Design review of the part shown in the three views and the two pictorial views. Dimensions are in mm from the part's minimum x, y and z. A direction names the side the tool comes from. Give positions to 0.01 mm unless a question says otherwise; leave off trailing zeros. Order: outer loops, then holes, each group sorted by start corner. A loop starts at its lowest first (then second) coordinate and runs counter-clockwise, first axis right, second up. Notation, with made-up numbers: (-3, -7.5) -> (22, -7.5) arc R20 cw to (22, 9.5) -> close; hole circle Ø1 at (61, 77.5). An arc over 180 degrees is marked (long way). Use one line per item in the form item = value.
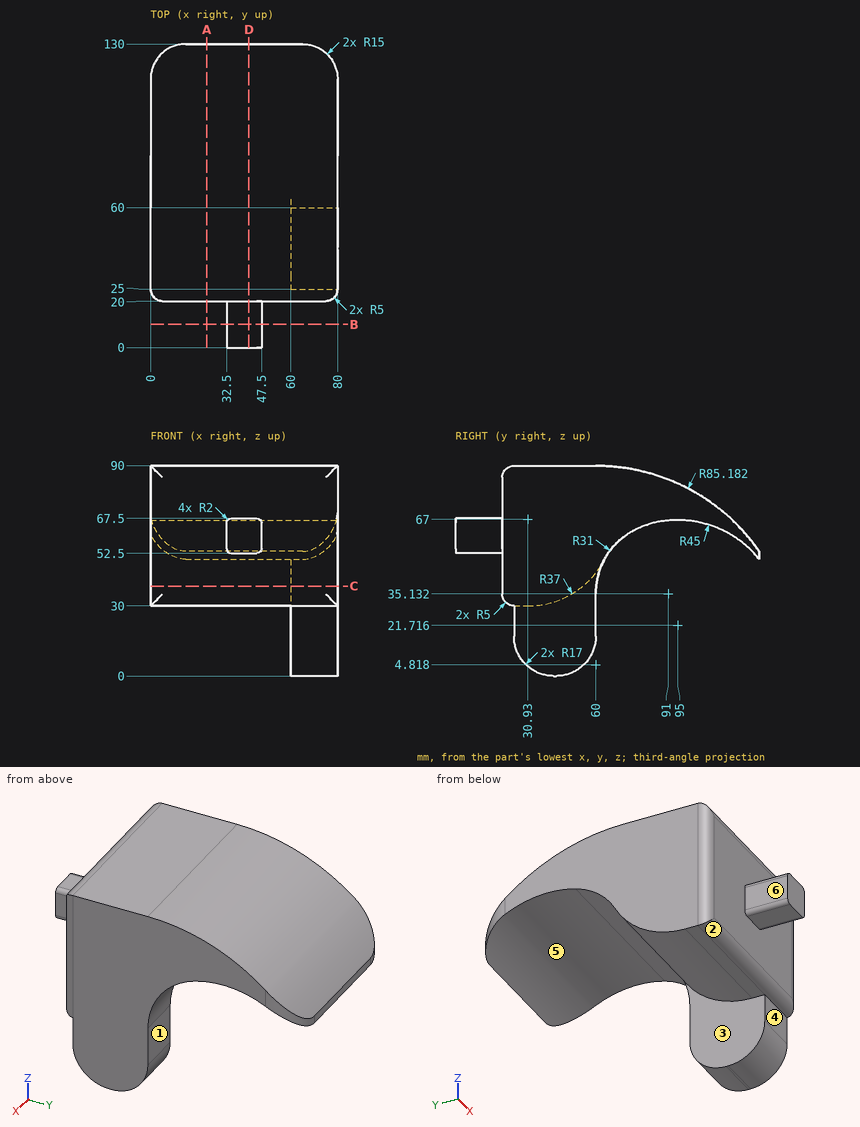
1. Add section C-C on z = 38.5. Give the boundary of the cut face in (x, y) (1 decimal), then the cut area to 3 significant figures.
Values:
outline = (0, 25) arc R5 ccw to (5, 20) -> (75, 20) arc R5 ccw to (80, 25) -> (80, 60.2) -> (60, 60.2) -> (60, 54.5) -> (0, 54.5) -> close
area = 2,860 mm^2
2. Add section B-B on y = 10. Give the boundary of the cut face in (x, z), then the cut area to 3 significant figures.
Values:
outline = (32.5, 54.5) arc R2 ccw to (34.5, 52.5) -> (45.5, 52.5) arc R2 ccw to (47.5, 54.5) -> (47.5, 65.5) arc R2 ccw to (45.5, 67.5) -> (34.5, 67.5) arc R2 ccw to (32.5, 65.5) -> close
area = 222 mm^2
3. Add section A-A on x = 24. Give the boundary of the cut face in (y, z) (1 decimal), then the cut area to 4 significant figures.
Values:
outline = (20, 35) arc R5 ccw to (25, 30) -> (30.9, 30) arc R37 ccw to (63.6, 49.7) arc R31 cw to (82.1, 64.8) arc R45 cw to (130, 50) -> (130, 53.4) arc R85.2 ccw to (60, 90) -> (25, 90) arc R5 ccw to (20, 85) -> close
area = 3,525 mm^2
4. Tool access review of the marked faces 1, 2 and 3: name each direction out of +Z, -Z, +X, -X, +Y, -Y from which nothing blocks a thin tool from reaching the whole face with its end or side.
Values:
face_1 = -Z, +X, -X, +Y
face_2 = -Z, +X, -X, -Y
face_3 = -Z, -X, +Y
5. For pin 1 Ø4 at (x, z) = (69, 21.5) entering from -Y; pin 2 Ø12 at (x, z) = (9.5, 66.5) entering from +Y; pin 3 Ø5 at (x, y) = (58.5, 95) entering from -Z, all flat-tipped, find the tip position at first contact; note any pin that passes through.
Values:
pin_1 = 25
pin_2 = 124.46
pin_3 = 66.65
6. For L1, parallel to Y at x = 54, z = 50.5; L2, parallel to X at y = 37, z = 23; L3, parallel to Z at x = 39.5, y = 31.5 (1 decimal), list the stretches that pass through material, from the lowest coordinate up.
Values:
L1 = 20 to 64.08, 129.59 to 130
L2 = 60 to 80
L3 = 30 to 90
7. Add section D-D on x = 42. Give the boundary of the cut face in (y, z) (1 decimal), then the cut area to 4 significant figures.
Values:
outline = (0, 52.5) -> (20, 52.5) -> (20, 35) arc R5 ccw to (25, 30) -> (30.9, 30) arc R37 ccw to (63.6, 49.7) arc R31 cw to (82.1, 64.8) arc R45 cw to (130, 50) -> (130, 53.4) arc R85.2 ccw to (60, 90) -> (25, 90) arc R5 ccw to (20, 85) -> (20, 67.5) -> (0, 67.5) -> close
area = 3,825 mm^2
8. The part is to be moulded in two halves that separate along Y. For the marked faces 4, 5 and 6, say which applies: +Y half, -Y half, draft (parallel to the pull), parting line (faces both ways), or undercut.
Values:
face_4 = -Y half
face_5 = undercut
face_6 = draft
